Part model, mm, in its own coordinate system. A direction names the side the tool comes from. Coordinates: 2 decimals unless noted, no trailing zeros. Order: outer loops, then holes, each group sorted by start corner. A loop starts at its lowest first (then second) coordinate and runs counter-clockwise, first axis right, second up. Notation, with made-up numbers: (12, -19.5) - (66, -19.5) arc R17 ccw to (66, -8.5) - close; hole circle Ø1 at (42.25, 6.25). An arc over 180 degrees is marked (long way). Use a Markdown table: item, result. Add a question column.
1) Drop flat-ended pins along their axis: P1, Ø10, axis at y = 69, z = -2.5, coming from the -X side; P2, Ø2.5, axis at x = -0.5, y = 61, coming from the +Z side; P3, Ø2.5, axis at x = 0.5, y = 68, coming from the -Z side. Give the stop position or say it passes through.
2) Wall check: L1, parallel to Z at x = 0, y = 45; L2, parallel to X at y = 59, z = 8; L3, parallel to Z at x = 4, y = 30. Give the ranges that are in metal, low to high. Write a range as [from, to].
3) Saw through at B-B on x = 0. List the corners of the cut face in (y, z).
4) Two-plate mould, pull along Z, no slides. Class faces 1 (the face through (-9, 62, -15)), 2 (the face through (5.71, 61.62, -7.83)), 3 (the face through (-4, 0, 0)): +Z half, -Z half, draft (parallel to the pull), parting line (faces both ways), or undercut.
5) Saw through at A-A on z = 0. List the corners of the cut face in (x, y).
6) Tool access for faces 4 (the face through (-5, 62, 0)), 5 (the face through (9, 62, -15)), 6 (the face through (-12, 62, 6)): list every direction of +Z, -Z, +X, -X, +Y, -Y with a clear straight run to the whole face (end or side of a thin tool).
```python
from build123d import *

# Parameters (mm, degrees)
F0_R     = 2
F1_DEPTH = 125


with BuildPart() as f1:
    # F0 (on Front) → F1 (new body)
    with BuildSketch(Plane.XZ):
        with BuildLine():
            ThreePointArc((15, 13.5), (14.56066, 14.56066), (13.5, 15))
            Line((13.5, 15), (4, 15))
            ThreePointArc((4, 15), (3.292893, 14.707107), (3, 14))
            Line((3, 14), (3, 13))
            ThreePointArc((3, 13), (3.292893, 12.292893), (4, 12))
            Line((4, 12), (7.464466, 12))
            ThreePointArc((7.464466, 12), (8.388346, 11.382683), (8.171573, 10.292893))
            Line((8.171573, 10.292893), (3.318019, 5.43934))
            ThreePointArc((3.318019, 5.43934), (2.831384, 5.114181), (2.257359, 5))
            Line((2.257359, 5), (-2.257359, 5))
            ThreePointArc((-2.257359, 5), (-2.831384, 5.114181), (-3.318019, 5.43934))
            Line((-3.318019, 5.43934), (-8.171573, 10.292893))
            ThreePointArc((-8.171573, 10.292893), (-8.388346, 11.382683), (-7.464466, 12))
            Line((-7.464466, 12), (-4, 12))
            ThreePointArc((-4, 12), (-3.292893, 12.292893), (-3, 13))
            Line((-3, 13), (-3, 14))
            ThreePointArc((-3, 14), (-3.292893, 14.707107), (-4, 15))
            Line((-4, 15), (-13.5, 15))
            ThreePointArc((-13.5, 15), (-14.56066, 14.56066), (-15, 13.5))
            Line((-15, 13.5), (-15, 4))
            ThreePointArc((-15, 4), (-14.707107, 3.292893), (-14, 3))
            Line((-14, 3), (-13, 3))
            ThreePointArc((-13, 3), (-12.292893, 3.292893), (-12, 4))
            Line((-12, 4), (-12, 7.464466))
            ThreePointArc((-12, 7.464466), (-11.382683, 8.388346), (-10.292893, 8.171573))
            Line((-10.292893, 8.171573), (-5.43934, 3.318019))
            ThreePointArc((-5.43934, 3.318019), (-5.114181, 2.831384), (-5, 2.257359))
            Line((-5, 2.257359), (-5, -2.257359))
            ThreePointArc((-5, -2.257359), (-5.114181, -2.831384), (-5.43934, -3.318019))
            Line((-5.43934, -3.318019), (-10.292893, -8.171573))
            ThreePointArc((-10.292893, -8.171573), (-11.382683, -8.388346), (-12, -7.464466))
            Line((-12, -7.464466), (-12, -4))
            ThreePointArc((-12, -4), (-12.292893, -3.292893), (-13, -3))
            Line((-13, -3), (-14, -3))
            ThreePointArc((-14, -3), (-14.707107, -3.292893), (-15, -4))
            Line((-15, -4), (-15, -13.5))
            ThreePointArc((-15, -13.5), (-14.56066, -14.56066), (-13.5, -15))
            Line((-13.5, -15), (-4, -15))
            ThreePointArc((-4, -15), (-3.292893, -14.707107), (-3, -14))
            Line((-3, -14), (-3, -13))
            ThreePointArc((-3, -13), (-3.292893, -12.292893), (-4, -12))
            Line((-4, -12), (-7.464466, -12))
            ThreePointArc((-7.464466, -12), (-8.388346, -11.382683), (-8.171573, -10.292893))
            Line((-8.171573, -10.292893), (-3.318019, -5.43934))
            ThreePointArc((-3.318019, -5.43934), (-2.831384, -5.114181), (-2.257359, -5))
            Line((-2.257359, -5), (2.257359, -5))
            ThreePointArc((2.257359, -5), (2.831384, -5.114181), (3.318019, -5.43934))
            Line((3.318019, -5.43934), (8.171573, -10.292893))
            ThreePointArc((8.171573, -10.292893), (8.388346, -11.382683), (7.464466, -12))
            Line((7.464466, -12), (4, -12))
            ThreePointArc((4, -12), (3.292893, -12.292893), (3, -13))
            Line((3, -13), (3, -14))
            ThreePointArc((3, -14), (3.292893, -14.707107), (4, -15))
            Line((4, -15), (13.5, -15))
            ThreePointArc((13.5, -15), (14.56066, -14.56066), (15, -13.5))
            Line((15, -13.5), (15, -4))
            ThreePointArc((15, -4), (14.707107, -3.292893), (14, -3))
            Line((14, -3), (13, -3))
            ThreePointArc((13, -3), (12.292893, -3.292893), (12, -4))
            Line((12, -4), (12, -7.464466))
            ThreePointArc((12, -7.464466), (11.382683, -8.388346), (10.292893, -8.171573))
            Line((10.292893, -8.171573), (5.43934, -3.318019))
            ThreePointArc((5.43934, -3.318019), (5.114181, -2.831384), (5, -2.257359))
            Line((5, -2.257359), (5, 2.257359))
            ThreePointArc((5, 2.257359), (5.114181, 2.831384), (5.43934, 3.318019))
            Line((5.43934, 3.318019), (10.292893, 8.171573))
            ThreePointArc((10.292893, 8.171573), (11.382683, 8.388346), (12, 7.464466))
            Line((12, 7.464466), (12, 4))
            ThreePointArc((12, 4), (12.292893, 3.292893), (13, 3))
            Line((13, 3), (14, 3))
            ThreePointArc((14, 3), (14.707107, 3.292893), (15, 4))
            Line((15, 4), (15, 13.5))
        make_face()
        Circle(F0_R, mode=Mode.SUBTRACT)
    extrude(amount=-F1_DEPTH)


solid = f1.part
```
Results are:
| question | item | result |
|---|---|---|
| 1 | P1 | x = -15 |
| 1 | P2 | z = 5 |
| 1 | P3 | z = -5 |
| 2 | L1 | [-5, -2], [2, 5] |
| 2 | L2 | [-15, -11.84], [-10.12, -5.88], [5.88, 10.12], [11.84, 15] |
| 2 | L3 | [-15, -12], [-6.12, 6.12], [12, 15] |
| 3 | outline | (0, -5) - (125, -5) - (125, -2) - (0, -2) - close; (0, 2) - (125, 2) - (125, 5) - (0, 5) - close |
| 4 | face 1 | -Z half |
| 4 | face 2 | undercut |
| 4 | face 3 | draft |
| 5 | outline | (-5, 0) - (-2, 0) - (-2, 125) - (-5, 125) - close; (2, 0) - (5, 0) - (5, 125) - (2, 125) - close |
| 6 | face 4 | -X, +Y, -Y |
| 6 | face 5 | -Z, +X, -X, +Y, -Y |
| 6 | face 6 | +Y, -Y |
